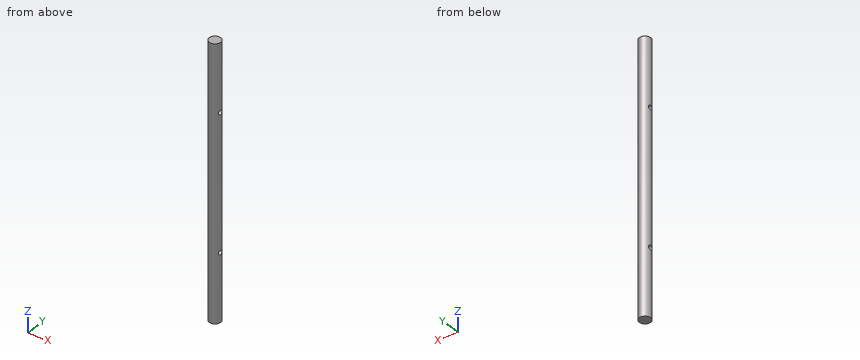
Autodesk Inventor part; units mm, degrees
ref_plane "YZ Plane" through (0, 0, 0) normal (1, 0, 0) x (0, 1, 0)
ref_plane "XZ Plane" through (0, 0, 0) normal (0, 1, 0) x (-1, 0, 0)
ref_plane "XY Plane" through (0, 0, 0) normal (0, 0, 1) x (1, 0, 0)
sketch "Sketch1" plane through (0, 0, 0) normal (1, 0, 0) x (0, 1, 0)
  line L0 (12.7, 300) -> (-12.7, 300)
  line L1 (-12.7, 300) -> (-12.7, -300)
  line L2 (-12.7, -300) -> (12.7, -300)
  line L3 (12.7, -300) -> (12.7, 300)
  line L4 (12.7, 300) -> (-12.7, -300) construction
  line L5 (-12.7, 300) -> (12.7, -300) construction
  circle A0 centre (0, 150) radius 5
  circle A1 centre (0, -150) radius 5
  line L6 (0, 0) -> (0, -150)
  dimension "d0" = 25.4
  dimension "d1" = 600
  dimension "d3" = 10
  dimension "d8" = 150
extrude "Extrusion1" add sketch "Sketch1" along normal blind 25.4
fillet "Fillet1" radius 12.7 4 edges at (25.4, -12.7, 0) (0, -12.7, 0) (25.4, 12.7, 0) (0, 12.7, 0)
properties part number "Eixo_traseiro"
Geometry: final body of the model. Coordinates: model frame, mm. Coordinates: 2 decimals unless noted, no trailing zeros. Order: outer loops, then holes, each group sorted by start corner. A loop starts at its lowest first (then second) coordinate and runs counter-clockwise, first axis right, second up. Notation, with made-up numbers: (-14.75, 8.25) -> (19.25, 8.25) arc R20 cw to (19.25, 14.25) -> close; hole circle Ø10 at (-11, 43.25). An arc over 180 degrees is marked (long way). Write item = value, one per line.
(1) Line query: line 1 (Z direction, x = 13.75, y = 0); line 2 (Z direction, x = 3, y = -1.5); line 3 (Y direction, x = 14.25, z = -150). Output: solid intervals per line, ascending.
Solved:
line_1 = -300 to -155, -145 to 145, 155 to 300
line_2 = -300 to -154.77, -145.23 to 145.23, 154.77 to 300
line_3 = -12.61 to -5, 5 to 12.61
(2) Cut plane C-C on z = -150. Return loops of the section in (x, y).
Solved:
outline = (1.03, -5) arc R12.7 ccw to (24.37, -5) -> close; (1.03, 5) -> (24.37, 5) arc R12.7 ccw to start
(3) Cut plane D-D on z = 223. Return loops of the section in (x, y), plus the area to 3 significant figures.
Solved:
outline = circle Ø25.4 at (12.7, 0)
area = 507 mm²
(4) Cut plane B-B on x = 8.5. Return loops of the section in (y, z).
Solved:
outline = (-11.99, -300) -> (11.99, -300) -> (11.99, 300) -> (-11.99, 300) -> close; hole circle Ø10 at (0, -150); hole circle Ø10 at (0, 150)
(5) Cut plane A-A on y = 0. Return loops of the section in (x, z).
Solved:
outline = (0, -300) -> (25.4, -300) -> (25.4, -155) -> (0, -155) -> close; (0, -145) -> (25.4, -145) -> (25.4, 145) -> (0, 145) -> close; (0, 155) -> (25.4, 155) -> (25.4, 300) -> (0, 300) -> close
(6) Pin query (flat end, axial travel): pin 1 Ø12 at (y, z) = (-7, -194.5) entering from -X; pin 2 Ø6 at (y, z) = (0, 150) entering from +X; pin 3 Ø1 at (x, z) = (12, -53) entering from -Y; pin 4 Ø6 at (y, z) = (-5, 66) entering from +X. Return the tip coordinate at first contact, or that it passes through.
Solved:
pin_1 = 0.04
pin_2 = through
pin_3 = -12.7
pin_4 = 25.24
